Autodesk Inventor part; units mm, degrees
ref_plane "YZ Plane" through (0, 0, 0) normal (1, 0, 0) x (0, 1, 0)
ref_plane "XZ Plane" through (0, 0, 0) normal (0, 1, 0) x (-1, 0, 0)
ref_plane "XY Plane" through (0, 0, 0) normal (0, 0, 1) x (1, 0, 0)
sketch "Sketch1" plane through (0, 0, 0) normal (0, 0, 1) x (1, 0, 0)
  line L0 (-10, -10) -> (-5.6, -10)
  line L1 (-10, -5.6) -> (-10, -10)
  line L2 (-5.6, -10) -> (-5, -10)
  line L3 (-3.2, -8.2) -> (-5.6, -8.2)
  line L4 (-2.8351, -3.825) -> (-5.6, -6.5899)
  line L5 (-3.825, -2.8351) -> (-6.5899, -5.6)
  line L6 (0, 0) -> (0, -11) construction
  line L7 (0, 0) -> (-12, 0) construction
  line L8 (-3.2, -8.2) -> (-5, -10)
  line L9 (-6.5899, -5.6) -> (-8.2, -5.6)
  line L10 (-10, -5.6) -> (-10, -5)
  line L11 (-10, -5) -> (-8.2, -3.2)
  line L12 (-8.2, -3.2) -> (-8.2, -5.6)
  line L13 (-5.6, -8.2) -> (-5.6, -6.5899)
  arc A0 (-2.15, 0) -> (0, -2.15) centre (0, 0) ccw
  line L14 (0, 0) -> (-3.825, 0)
  line L15 (-3.825, 0) -> (-3.825, -2.8351)
  line L16 (-2.8351, -3.825) -> (0, -3.825)
  line L17 (0, -3.825) -> (0, 0)
  line L18 (-2.8351, -3.825) -> (-3.825, -3.825) construction
  line L19 (-3.825, -3.825) -> (-3.825, -2.8351) construction
  line L20 (3.825, -2.8351) -> (3.825, -3.825) construction
  line L21 (3.825, -2.8351) -> (3.825, 0)
  line L22 (3.825, -3.825) -> (2.8351, -3.825) construction
  line L23 (3.825, 0) -> (0, 0)
  line L24 (0, -3.825) -> (2.8351, -3.825)
  arc A1 (0, -2.15) -> (2.15, 0) centre (0, 0) ccw
  line L25 (0, 0) -> (0, -3.825)
  line L26 (2.8351, -3.825) -> (5.6, -6.5899)
  line L27 (0, 0) -> (0, -12) construction
  line L28 (0, 0) -> (11, 0) construction
  line L29 (3.825, -2.8351) -> (6.5899, -5.6)
  line L30 (8.2, -3.2) -> (8.2, -5.6)
  line L31 (10, -5.6) -> (10, -5)
  line L32 (8.2, -3.2) -> (10, -5)
  line L33 (8.2, -5.6) -> (6.5899, -5.6)
  line L34 (5.6, -6.5899) -> (5.6, -8.2)
  line L35 (10, -10) -> (10, -5.6)
  line L36 (5.6, -10) -> (10, -10)
  line L37 (3.2, -8.2) -> (5.6, -8.2)
  line L38 (5, -10) -> (3.2, -8.2)
  line L39 (5.6, -10) -> (5, -10)
  line L40 (2.8351, 3.825) -> (3.825, 3.825) construction
  line L41 (2.8351, 3.825) -> (0, 3.825)
  line L42 (3.825, 3.825) -> (3.825, 2.8351) construction
  line L43 (0, 3.825) -> (0, 0)
  line L44 (3.825, 0) -> (3.825, 2.8351)
  arc A2 (2.15, 0) -> (0, 2.15) centre (0, 0) ccw
  line L45 (0, 0) -> (3.825, 0)
  line L46 (3.825, 2.8351) -> (6.5899, 5.6)
  line L47 (0, 0) -> (12, 0) construction
  line L48 (0, 0) -> (0, 11) construction
  line L49 (2.8351, 3.825) -> (5.6, 6.5899)
  line L50 (3.2, 8.2) -> (5.6, 8.2)
  line L51 (5.6, 10) -> (5, 10)
  line L52 (3.2, 8.2) -> (5, 10)
  line L53 (5.6, 8.2) -> (5.6, 6.5899)
  line L54 (6.5899, 5.6) -> (8.2, 5.6)
  line L55 (10, 10) -> (5.6, 10)
  line L56 (10, 5.6) -> (10, 10)
  line L57 (8.2, 3.2) -> (8.2, 5.6)
  line L58 (10, 5) -> (8.2, 3.2)
  line L59 (10, 5.6) -> (10, 5)
  line L60 (-3.825, 2.8351) -> (-3.825, 3.825) construction
  line L61 (-3.825, 2.8351) -> (-3.825, 0)
  line L62 (-3.825, 3.825) -> (-2.8351, 3.825) construction
  line L63 (-3.825, 0) -> (0, 0)
  line L64 (0, 3.825) -> (-2.8351, 3.825)
  arc A3 (0, 2.15) -> (-2.15, 0) centre (0, 0) ccw
  line L65 (0, 0) -> (0, 3.825)
  line L66 (-2.8351, 3.825) -> (-5.6, 6.5899)
  line L67 (0, 0) -> (0, 12) construction
  line L68 (0, 0) -> (-11, 0) construction
  line L69 (-3.825, 2.8351) -> (-6.5899, 5.6)
  line L70 (-8.2, 3.2) -> (-8.2, 5.6)
  line L71 (-10, 5.6) -> (-10, 5)
  line L72 (-8.2, 3.2) -> (-10, 5)
  line L73 (-8.2, 5.6) -> (-6.5899, 5.6)
  line L74 (-5.6, 6.5899) -> (-5.6, 8.2)
  line L75 (-10, 10) -> (-10, 5.6)
  line L76 (-5.6, 10) -> (-10, 10)
  line L77 (-3.2, 8.2) -> (-5.6, 8.2)
  line L78 (-5, 10) -> (-3.2, 8.2)
  line L79 (-5.6, 10) -> (-5, 10)
  point P0 (0, 2.15)
  point P1 (2.15, 0)
  point P2 (0, -2.15)
  dimension "d16" = 10
  dimension "d19" = 3.2
  dimension "d21" = 4.4
  dimension "d22" = 4.4
  dimension "d24" = 45
  dimension "d25" = 1.8
  dimension "d27" = 1.8
  dimension "d28" = 45
  dimension "d29" = 3.2
  dimension "d31" = 1.4
  dimension "d33" = 2.15
  dimension "d34" = 3.825
  dimension "d35" = 3.825
  dimension "d36" = 135
  dimension "d39" = 360
extrude "Extrusion1" add sketch "Sketch1" along normal blind 360 contours L1 L10 L11 L12 L9 L5 L15 L14 A0 L17 L16 L4 L13 L3 L8 L2 L0 | L17 A1 L23 L21 L29 L33 L30 L32 L31 L35 L36 L39 L38 L37 L34 L26 L24 | L61 L69 L73 L70 L72 L71 L75 L76 L79 L78 L77 L74 L66 L64 L43 A3 L14 | A2 L43 L41 L49 L53 L50 L52 L51 L55 L56 L59 L58 L57 L54 L46 L44 L23
pattern_linear "Rectangular Pattern1" count 2 spacing 20 along (0, -1, 0) of "Extrusion1"
sketch "Sketch2" plane through (0, 0, 360) normal (0, 0, 1) x (1, 0, 0)
  line L0 (3.2, -8.2) -> (5, -10)
  line L1 (-3.2, -11.8) -> (-5, -10)
  line L2 (5, -10) -> (-5, -10) construction
  line L3 (-8.2, -12.25) -> (8.2, -12.25)
  line L4 (8.2, -12.25) -> (8.2, -7.75)
  line L5 (8.2, -7.75) -> (-8.2, -7.75)
  line L6 (-8.2, -7.75) -> (-8.2, -12.25)
  line L7 (-8.2, -12.25) -> (8.2, -7.75) construction
  line L8 (8.2, -12.25) -> (-8.2, -7.75) construction
  line L9 (10, -15) -> (10, -5)
  line L10 (5.6, -6.5899) -> (5.6, -8.2)
  line L11 (5.6, -6.5899) -> (6.7601, -7.75)
  line L12 (-5.6, -6.5899) -> (-2.8351, -3.825)
  line L13 (-5.6, -6.5899) -> (-6.7601, -7.75)
  line L14 (5.6, -13.4101) -> (6.7601, -12.25)
  line L15 (-5.6, -13.4101) -> (-6.7601, -12.25)
  line L16 (-5.6, -6.5899) -> (-5.6, -7.75)
  line L17 (-5.6, -8.2) -> (-5.6, -6.5899)
  line L18 (5.6, -6.5899) -> (5.6, -7.75)
  line L19 (-5.6, -11.8) -> (-5.6, -13.4101)
  line L20 (5.6, -13.4101) -> (5.6, -12.25)
  point P0 (0, 0)
  point P1 (0, -10)
  point P2 (-5.6, -12.25)
  dimension "d46" = 4.5
  dimension "d50" = 1.8
extrude "Extrusion2" cut sketch "Sketch2" against normal blind 400
properties part number "AP20x20"
Input: part model. Units: mm. Frame: model coordinates. A direction names the side the tool comes from. Give positions to 0.01 mm unless a question says otherwise; leave off trailing zeros. Write each question's results on one line, items separated by ' | '. Start each with the question number.
Item 1: Set-up query: faces 1 (the flat face through (0, -3.825, 177)), 2 (the flat face through (3.825, -20, 177)), 3 (the flat face through (0, -23.825, 177)), 4 (the flat face through (-3.825, -20, 177)), 5 (the flat face through (0, 3.825, 177)). Return all of +Z, -Z, +X, -X, +Y, -Y with unobstructed straight access to the full face (end or side cutting, diameter ignored); none if empty.
Item 2: Line query: line 1 (Y direction, x = 0, z = 253.5) (3 decimals); line 2 (Y direction, x = 7.75, z = 74.5); line 3 (Y direction, x = -2.75, z = 311) (3 decimals). Output: solid intervals per line, ascending.
Item 3: Mould query, pull axis X, two halves, no side actions, for faces 6 (the flat face through (-10, -10, 177)), 7 (the flat face through (3.825, 0, 177)), 8 (the flat face through (0, -16.175, 177)). Classes: pulls with the +X half, pulls with the -X half, needs draft (parallel to the pull), parting line crosses it, or undercut.
Item 4: Contact query for flat-ended pins moving along their axis: P1, Ø1, axis at x = 1, z = 178.5, coming from the -Y side (3 decimals); P2, Ø1.5, axis at x = 0.5, z = 271.5, coming from the +Y side (3 decimals); P3, Ø6, axis at y = -21.5, z = 284.5, coming from the -X side. Output: stop coordinate, or through.
Item 5: Cut plane A-A on z = 325. Give the number of separate pieces and of enclosed holes in the cut face, then the cut area to 3 significant figures.
Established:
1) face 1: +Z, -Z | face 2: +Z, -Z, +X | face 3: +Z, -Z, -Y | face 4: +Z, -Z, -X | face 5: +Z, -Z, +Y
2) line 1: -23.825 to -22.15, -17.85 to -16.175, -3.825 to -2.15, 2.15 to 3.825 | line 2: -30 to -25.6, -14.4 to -12.25, -7.75 to -5.6, 5.6 to 10 | line 3: -23.825 to -16.175, -3.825 to 3.825
3) face 6: pulls with the -X half | face 7: pulls with the +X half | face 8: undercut
4) P1: y = -23.825 | P2: y = 3.825 | P3: x = -9.5
5) separate pieces: 1 | enclosed holes: 3 | area: 285 mm^2
